Read the model definition and answer for the solid it produces. Units are mm, in the model's axes. Face numbers are marked on the shaded views. A direction names the side the tool comes from. Round coordinates to 2 decimals unless told otherwise and drop trailing zeros. Order: outer loops, then holes, each group sorted by start corner. A loop starts at its lowest first (then second) coordinate and runs counter-clockwise, first axis right, second up. Notation, with made-up numbers: (14.25, -39.5) - (18.25, -39.5) arc R27 cw to (18.25, -11.5) - close; hole circle Ø8 at (-40, 82.25). An arc over 180 degrees is marked (long way). Answer as a JSON object with one key per item and string values. Group by question number.
Q1. The mould has two halves that part along Y. Classify the marked faces 4, 5 and 6: pulls with the +Y half, pulls with the -Y half, needs draft (parallel to the pull), parting line crosses it, or undercut.
Q2. A cutting plane is placed at B-B on x = -57.5. Determine the outline of the cut face in (y, z), and give its area (3 significant figures).
Q3. A tool of negligible diameter and unlimited length cuts with its end or side. For the marked faces 1, 2 and 3, from which of +Z, -Z, +X, -X, +Y, -Y can it reach the whole face along a straight path? Write none if from no direction.
Q4. Given pin 1 Ø3 at (x, z) = (-37, -14.5) entering from -Y; pin 2 Ø1.5 at (x, z) = (-52.5, 39.5) entering from +Y; pin 3 Ø12 at (x, y) = (-68.5, -25) entering from -Z, each flat-ended and moving along its own axis, determine where each tip first touches the part or whether it passes through.
Q5. A cutting plane is placed at A-A on x = -7.5. Determine the outline of the cut face in (y, z), and give its area (3 significant figures).
Q6. Consider line 1 (Y direction, x = -10.25, z = 0); line 2 (X direction, y = -17.5, z = 56.5); line 3 (Y direction, x = -62, z = 0). Determine where each line is inside the solid, lowest interval first.
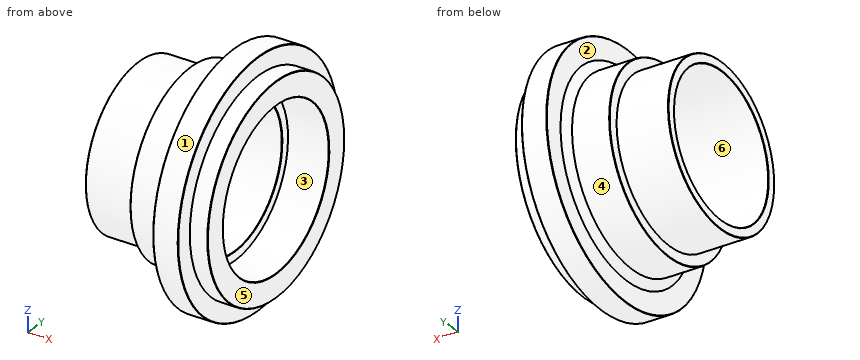
```python
from build123d import *

# Parameters (mm, degrees)
CHANFREIN1_SIZE = 0.2
CHANFREIN2_SIZE = 0.2


with BuildPart() as part:
    # Esquisse1 → Révolution1 (revolve)
    with BuildSketch(Plane.XY, mode=Mode.PRIVATE) as r_volution1_sk:
        Polygon((0, 45), (0, 58), (-10, 58), (-10, 68), (-24, 68), (-24, 56.196152423), (-27, 51), (-48, 51), (-48, 45), (-77, 45), (-77, 40), (-23, 40), (-23, 45), align=None)
    revolve(r_volution1_sk.sketch.rotate(Axis((0, 0, 0), (-1, 0, 0)), 90), axis=Axis((0, 0, 0), (-1, 0, 0)))  # turned: the seam where the file's is

    # Chanfrein1
    chanfrein1_edges = [part.edges().sort_by_distance(p)[0] for p in [
        (-48, 0, 51),
        (-77, 0, 45),
        (-77, 0, 40),
        (0, 0, 45),
        (0, 0, 58),
        (-10, 0, 68),
        (-24, 0, 68),
    ]]
    chamfer(chanfrein1_edges, length=CHANFREIN1_SIZE)

    # Chanfrein2
    chanfrein2_edges = [part.edges().sort_by_distance(p)[0] for p in [
        (-23, 0, 40),
    ]]
    chamfer(chanfrein2_edges, length=CHANFREIN2_SIZE)


solid = part.part
```
Result set:
{
 "1": {"face 4": "parting line crosses it", "face 5": "needs draft", "face 6": "undercut"},
 "2": {"outline": "circle Ø90 at (0, 0); hole circle Ø80 at (0, 0)", "area": "1,340 mm²"},
 "3": {"face 1": "+X, -X", "face 2": "-X", "face 3": "+X"},
 "4": {"pin 1": "stops at y = -49.32", "pin 2": "stops at y = 22.88", "pin 3": "stops at z = -40.79"},
 "5": {"outline": "circle Ø116 at (0, 0); hole circle Ø90 at (0, 0)", "area": "4,210 mm²"},
 "6": {"line 1": "y = -68 to -45, 45 to 68", "line 2": "x = -24 to -10", "line 3": "y = -45 to -40, 40 to 45"}
}
